```python
from build123d import *

# Parameters (mm, degrees)
F1_DEPTH = 12.7
F2_SIZE  = 4.572


# Not quite as in the source:
# - a feature names something its author has since deleted; it is built from what else it names


with BuildPart() as f1:
    # F0 (on Top) → F1 (new body)
    with BuildSketch(Plane.XY):
        Polygon((-138.7197226286, 19.6580234915), (-180.3987026215, -27.6248455048), (-85.8329609036, 8.0999890342), (-97.3909944296, -18.1682743132), (-23.6561261117, 16.663254671), (-23.6561261117, -9.9510056898), (0, 14.3561139703), (18.1893575937, 49.4287200272), (-20.6876713783, 39.6219007671), (-9.3052154407, 49.093272537), (-60.4820251465, 49.093272537), (-72.0571577549, 39.281655103), (-138.0494087934, 38.2558703423), (-124.7141808271, 59.4554506242), (-153.0797034502, 94.610132277), (-136.6182565689, 96.7115908861), (-189.1547888517, 134.5378756523), (-165.3382331133, 69.3925991654), (-178.2972365618, 25.9624067694), align=None)
    extrude(amount=F1_DEPTH)

    # F2
    f2_edges = [f1.edges().sort_by_distance(p)[0] for p in [
        (-162.886523, 115.624733, 12.7),
        (-177.246511, 101.965237, 12.7),
        (-171.817735, 47.677503, 12.7),
        (-158.50848, 22.810215, 12.7),
        (-159.559213, -3.983411, 12.7),
        (-133.115832, -9.762428, 12.7),
        (-91.611978, -5.034143, 12.7),
        (-60.52356, -0.75251, 12.7),
        (-23.656126, 3.356124, 12.7),
        (-11.828063, 2.202554, 12.7),
        (9.094679, 31.892417, 12.7),
        (-1.249157, 44.52531, 12.7),
        (-14.996443, 44.357587, 12.7),
        (-34.89362, 49.093273, 12.7),
        (-66.269591, 44.187464, 12.7),
        (-105.053283, 38.768763, 12.7),
        (-131.381795, 48.85566, 12.7),
        (-138.896942, 77.032791, 12.7),
        (-144.84898, 95.660862, 12.7),
    ]]
    chamfer(f2_edges, length=F2_SIZE)


solid = f1.part
```
Design review of the part built by this model. Coordinates are the model's own, in mm. A direction names the side the tool comes from. Coordinates: 2 decimals unless noted, no trailing zeros. Write each loop counter-clockwise with the first axis right and the second up, starting at its lowest first coordinate (ties: lowest second). Pieces come first, ordered by that corner, then holes. Notation, with made-up numbers: M 13,-11.75 L 40,-11.75 A11 ccw 40,-4.75 Z; hole C 88.5,65.5 d9. An arc over 180 degrees is marked long. Answer as a JSON object with one key per item and string values.
Item 1: Add section A-A, the plane z = 4. Give the boundary of the cut face in (x, y).
Outcome:
{"outline": "M -189.15,134.54 L -165.34,69.39 L -178.3,25.96 L -138.72,19.66 L -180.4,-27.62 L -85.83,8.1 L -97.39,-18.17 L -23.66,16.66 L -23.66,-9.95 L 0,14.36 L 18.19,49.43 L -20.69,39.62 L -9.31,49.09 L -60.48,49.09 L -72.06,39.28 L -138.05,38.26 L -124.71,59.46 L -153.08,94.61 L -136.62,96.71 Z"}
Item 2: Wall thickness on probe 1 along Y at (x, z) = (-139.5, 1.75); probe 2 along Y at (x, z) = (-153.5, 8.25); probe 3 along X at (y, z) = (17, 11.5): over which ranges is each line inside the solid? List them lowest first.
Outcome:
{"probe 1": "-12.17 to 18.77, 19.78 to 77.78, 96.34 to 98.79", "probe 2": "-17.33 to 2.71, 22.14 to 108.72", "probe 3": "-136.57 to -30.84, -20.28 to -2.43"}
Item 3: Add section C-C, the plane y = 63. Give the boundary of the cut face in (x, z).
Outcome:
{"outline": "M -167.25,0 L -127.57,0 L -127.57,8.13 L -133.45,12.7 L -162.47,12.7 L -167.25,8.13 Z"}
Item 4: Insertion check: pin 1 Ø2 at (x, z) = (-56.5, 10) entering from +Y; pin 2 Ø3 at (x, z) = (-78, 2) entering from -Y; pin 3 Ø1.5 at (x, z) = (-108.5, 9) entering from +Y. Each pin has a flat end and moves straight along its axis. Give the tip position at first contact, or say it passes through.
Outcome:
{"pin 1": "y = 48.22", "pin 2": "y = -9.72", "pin 3": "y = 38.59"}
Item 5: Add section B-B, the plane x = -108. Give the boundary of the cut face in (y, z), and give its area (3 significant figures).
Outcome:
{"outline": "M -0.27,0 L 38.72,0 L 38.72,8.13 L 34.15,12.7 L 4.61,12.7 L -0.27,8.13 Z", "area": "474 mm²"}
Item 6: Machinability: for faces 1 (the flat face through (-154.74, -2.03, 10.45)), 2 (the flat face through (-58.813, 2.619, 10.446)), 3 (the flat face through (-24.4, 39.55, 10.45)), 4 (the flat face through (-158.786, 22.854, 4.007)), 5 (the flat face through (-143, 78.5, 10.4)), which of the approach directions +Z, -Z, +X, -X, +Y, -Y give a long, thin tool a straight path to every point of the face, cutting with its end or side? Answer none if there is none.
Outcome:
{"face 1": "+Z, -X", "face 2": "+Z, -Y", "face 3": "+Z", "face 4": "+Z, -Z, -X", "face 5": "+Z, +X"}
Item 7: Draft analysis for pull direction Y (two halves, no side actions). For faces 6 (the flat face through (-177.413, 102.421, 4.007)), 7 (the flat face through (-40.222, 46.775, 10.446)), 8 (the flat face through (-11.994, 2.032, 4.007)), state which applies: pulls with the +Y half, pulls with the -Y half, needs draft (parallel to the pull), parting line crosses it, or undercut.
Outcome:
{"face 6": "undercut", "face 7": "pulls with the +Y half", "face 8": "pulls with the -Y half"}
